Here's how the part is built. I have some questions about the finished solid (model axes, mm). A direction names the side the tool comes from. Give positions to 0.01 mm unless a question says otherwise; leave off trailing zeros. Loops run counter-clockwise (first coordinate to the right, second up) from the corner with the lowest first, then second, coordinate; pieces in that order, holes last. Notation, with made-up numbers: (73.5, 16) -> (80.5, 16) arc R19 cw to (80.5, 25) -> close; hole circle Ø10 at (68.25, 6.5). An arc over 180 degrees is marked (long way). Answer in a Markdown table with one row per item. Add a question column.
Item 1: If we section it at D-D (x = 13): Write out the boundary of the cut face in (y, z).
Item 2: We'd pull the mould along Z, two halves only. Please class faces 4 (the face through (-27.15, 2.96, 8)), 5 (the face through (-9, 15, 0)), 6 (the face through (-7.63, 15.48, -4)), 7 (the face through (15.1, 0.5, 2.5)): released by +Z, released by -Z, zero draft, split by the parting line, or undercut.
Item 3: If we section it at B-B (y = 2.5): Write out the boundary of the cut face in (x, z), then the cut area to 3 significant figures.
Item 4: Which directions (+Z, -Z, +X, -X, +Y, -Y) give clear straight access to the entire face, cutting with the end or side of a thin tool? Please do faces 1 (the face through (3.934, 15.479, -3.998)), 2 (the face through (3, 4, -3)), 3 (the face through (7.67, 15.48, -3.93)).
Item 5: If I drill on line 1 (Z direction, x = 0, y = 2.1); line 2 (Z direction, x = 0, y = 9.75); line 3 (Y direction, x = -3, z = -7.75), over which ranges is the centre line in solid material (lowest first)?
Item 6: For P1, Ø0.9, axis at y = 15, z = 0.5, coming from the -X side; P2, Ø5, axis at x = 0, z = 0, coming from the -Y side; P3, Ø5, axis at y = 2, z = 8.5, coming from the -X side, each with a flat end and sliding along its axis, tell me the tip position at first contact or that it passes through.
Item 7: If we section it at C-C (z = -7.5): Write out the boundary of the cut face in (x, y), then the cut area to 3 significant figures.
Item 8: If we section it at A-A (y = 15.25): Write out the boundary of the cut face in (x, z).
```python
from build123d import *

# Parameters (mm, degrees)
BOSS_EXTRUDE1_DEPTH                                 = 6
SKETCH2_R                                           = 11
BOSS_EXTRUDE2_DEPTH                                 = 8
SKETCH12_R                                          = 6
CUT_EXTRUDE2_DEPTH                                  = 4
BOSS_EXTRUDE3_DEPTH                                 = 3
CSK_FOR_M3_COUNTERSUNK_FLAT_HEAD_SCREW3_D           = 3.2
CSK_FOR_M3_COUNTERSUNK_FLAT_HEAD_SCREW3_CSINK_D     = 6.3
CSK_FOR_M3_COUNTERSUNK_FLAT_HEAD_SCREW3_CSINK_ANGLE = 90
CUT_EXTRUDE3_DEPTH                                  = 1


with BuildPart() as part:
    # Sketch1 → Boss-Extrude1 (new body)
    with BuildSketch(Plane(origin=(0, 0, 0), x_dir=(1, 0, 0), z_dir=(0, 1, 0))):
        with BuildLine():
            Line((-20.01, -11), (20.01, -11))
            ThreePointArc((20.01, -11), (27.073996744, -8.073996744), (30, -1.01))
            Line((30, -1.01), (30, 1.01))
            ThreePointArc((30, 1.01), (27.073996744, 8.073996744), (20.01, 11))
            Line((20.01, 11), (-20.01, 11))
            ThreePointArc((-20.01, 11), (-27.073996744, 8.073996744), (-30, 1.01))
            Line((-30, 1.01), (-30, -1.01))
            ThreePointArc((-30, -1.01), (-27.073996744, -8.073996744), (-20.01, -11))
        make_face()
    extrude(amount=BOSS_EXTRUDE1_DEPTH)

    # Sketch2 → Boss-Extrude2 (add)
    with BuildSketch(Plane(origin=(0, 6, 0), x_dir=(1, 0, 0), z_dir=(0, 1, 0))):
        Circle(SKETCH2_R)
    extrude(amount=BOSS_EXTRUDE2_DEPTH)

    # Sketch12 → Cut-Extrude2 (cut)
    with BuildSketch(Plane.XZ):
        Circle(SKETCH12_R)
    extrude(amount=-CUT_EXTRUDE2_DEPTH, mode=Mode.SUBTRACT)

    # Sketch19 → Boss-Extrude3 (add)
    with BuildSketch(Plane(origin=(0, 14, 0), x_dir=(1, 0, 0), z_dir=(0, 1, 0))):
        Polygon((-6.300393599, 6.426899758), (-9, 1.5), (-9, -1.5), (-6.300393599, -6.426899758), (-1.5, -1.5), (1.5, -1.5), (6.300393599, -6.426899758), (9, -1.5), (9, 1.5), (6.300393599, 6.426899758), (1.5, 1.5), (-1.5, 1.5), align=None)
    extrude(amount=BOSS_EXTRUDE3_DEPTH)

    # CSK for M3 Countersunk Flat Head Screw3 (through all)
    with Locations(Plane(origin=(0, 4, 0), x_dir=(-1, 0, 0), z_dir=(0, -1, 0))):
        with Locations((0, 0)):
            CounterSinkHole(CSK_FOR_M3_COUNTERSUNK_FLAT_HEAD_SCREW3_D / 2, CSK_FOR_M3_COUNTERSUNK_FLAT_HEAD_SCREW3_CSINK_D / 2, counter_sink_angle=CSK_FOR_M3_COUNTERSUNK_FLAT_HEAD_SCREW3_CSINK_ANGLE)

    # Sketch20 → Cut-Extrude3 (cut)
    with BuildSketch(Plane.XZ):
        Polygon((10, 2.5), (10, -2.5), (20, -2.5), (20, -6), (26, 0), (20, 6), (20, 2.5), align=None)
    extrude(amount=-CUT_EXTRUDE3_DEPTH, mode=Mode.SUBTRACT)


solid = part.part
```
Recorded:
| question | item | result |
|---|---|---|
| 1 | outline | (0, -11) -> (6, -11) -> (6, 11) -> (0, 11) -> (0, 2.5) -> (1, 2.5) -> (1, -2.5) -> (0, -2.5) -> close |
| 2 | face 4 | released by +Z |
| 2 | face 5 | zero draft |
| 2 | face 6 | released by -Z |
| 2 | face 7 | undercut |
| 3 | outline | (-30, -1.01) arc R9.99 ccw to (-20.01, -11) -> (20.01, -11) arc R9.99 ccw to (30, -1.01) -> (30, 1.01) arc R9.99 ccw to (20.01, 11) -> (-20.01, 11) arc R9.99 ccw to (-30, 1.01) -> close; hole circle Ø12 at (0, 0) |
| 3 | area | 1,120 mm^2 |
| 4 | face 1 | -Z, +Y |
| 4 | face 2 | -Y |
| 4 | face 3 | -Z, +X, +Y |
| 5 | line 1 | z = -11 to -6, 6 to 11 |
| 5 | line 2 | z = -11 to -1.6, 1.6 to 11 |
| 5 | line 3 | y = 0 to 14 |
| 6 | P1 | stops at x = -9 |
| 6 | P2 | stops at y = 4.65 |
| 6 | P3 | stops at x = -28.66 |
| 7 | outline | (-27.6, 0) -> (27.6, 0) -> (27.6, 6) -> (8.05, 6) -> (8.05, 14) -> (-8.05, 14) -> (-8.05, 6) -> (-27.6, 6) -> close |
| 7 | area | 460 mm^2 |
| 8 | outline | (-9, -1.5) -> (-6.3, -6.43) -> (-1.5, -1.5) -> (-0.56, -1.5) arc R1.6 cw to (-0.56, 1.5) -> (-1.5, 1.5) -> (-6.3, 6.43) -> (-9, 1.5) -> close; (0.56, -1.5) -> (1.5, -1.5) -> (6.3, -6.43) -> (9, -1.5) -> (9, 1.5) -> (6.3, 6.43) -> (1.5, 1.5) -> (0.56, 1.5) arc R1.6 cw to start |
